Input: part model. Units: mm. Frame: model coordinates. Round coordinates to 2 decimals unless told otherwise and drop trailing zeros. Order: outer loops, then holes, each group sorted by start corner. A loop starts at its lowest first (then second) coordinate and runs counter-clockwise, first axis right, second up.
Item 1: Line query: L1, parallel to Y at x = -9.5, z = 1.4; L2, parallel to Y at x = 52, z = -0.8; L3, parallel to X at y = 3, z = -0.35. Output: solid intervals per line, ascending.
Item 2: Cut plane D-D on y = -9.5. Output: boundary loops of the cut face in (x, z).
Item 3: Cut plane A-A on y = 57. Output: boundary loops of the cut face in (x, z).
Item 4: First-contact query: pin 1 (6 mm diameter, centred on x = -52, y = 57, fed in from -Z); pin 2 (4 mm diameter, centred on x = -52, y = -57, fed in from -Z). Flat tips, straight axial feed; report the tip coordinate or a pass-through.
Item 5: Cut plane B-B on z = 1.2. Output: boundary loops of the cut face in (x, y), then the cut area to 3 significant figures.
Item 6: Cut plane C-C on x = 52. Output: boundary loops of the cut face in (y, z).
```python
from build123d import *

# Parameters (mm, degrees)
BOSS_EXTRUDE1_DEPTH         = 2
BOSS_EXTRUDE1_DEPTH_BACK    = 2
SKETCH1_W                   = 130
SKETCH1_H                   = 130
TAP_DRILL_FOR_M5X0_8_TAP1_D = 5
SKETCH5_W                   = 50
SKETCH5_H                   = 25
CUT_EXTRUDE2_DEPTH          = 20


with BuildPart() as part:
    # Sketch1 → Boss-Extrude1 (new, two sides: drawn at the far end of the back side and taken through both)
    with BuildSketch(Plane.XY.offset(-BOSS_EXTRUDE1_DEPTH_BACK)):
        Rectangle(SKETCH1_W, SKETCH1_H)
    extrude(amount=BOSS_EXTRUDE1_DEPTH + BOSS_EXTRUDE1_DEPTH_BACK)

    # Tap Drill for M5x0.8 Tap1 (through all)
    with Locations(Plane(origin=(0, 0, -2), x_dir=(-1, 0, 0), z_dir=(0, 0, -1))):
        with Locations((-52, 57), (52, 57), (52, -57), (-52, -57)):
            Hole(TAP_DRILL_FOR_M5X0_8_TAP1_D / 2)

    # Sketch5 → Cut-Extrude2 (cut)
    with BuildSketch(Plane(origin=(0, 0, -2), x_dir=(-1, 0, 0), z_dir=(0, 0, -1))):
        Rectangle(SKETCH5_W, SKETCH5_H)
    extrude(amount=-CUT_EXTRUDE2_DEPTH, mode=Mode.SUBTRACT)


solid = part.part
```
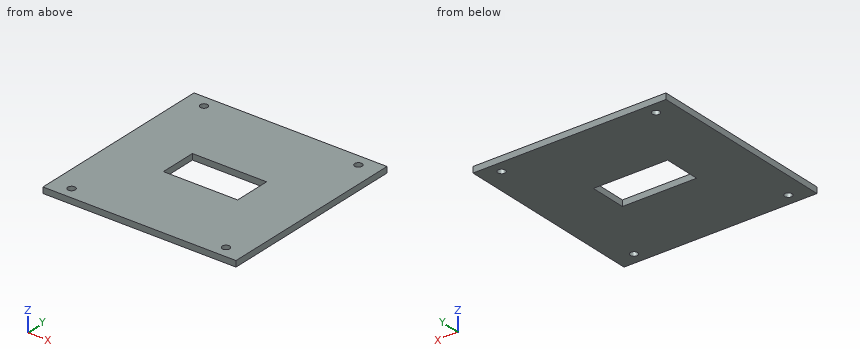
From the geometry:
1. L1: y = -65 to -12.5, 12.5 to 65
1. L2: y = -65 to -59.5, -54.5 to 54.5, 59.5 to 65
1. L3: x = -65 to -25, 25 to 65
2. outline: (-65, -2) - (-25, -2) - (-25, 2) - (-65, 2) - close; (25, -2) - (65, -2) - (65, 2) - (25, 2) - close
3. outline: (-65, -2) - (-54.5, -2) - (-54.5, 2) - (-65, 2) - close; (-49.5, -2) - (49.5, -2) - (49.5, 2) - (-49.5, 2) - close; (54.5, -2) - (65, -2) - (65, 2) - (54.5, 2) - close
4. pin 1: stops at z = -2
4. pin 2: passes through
5. outline: (-65, -65) - (65, -65) - (65, 65) - (-65, 65) - close; hole circle Ø5 at (-52, -57); hole circle Ø5 at (-52, 57); hole (-25, -12.5) - (25, -12.5) - (25, 12.5) - (-25, 12.5) - close; hole circle Ø5 at (52, -57); hole circle Ø5 at (52, 57)
5. area: 15,600 mm2
6. outline: (-65, -2) - (-59.5, -2) - (-59.5, 2) - (-65, 2) - close; (-54.5, -2) - (54.5, -2) - (54.5, 2) - (-54.5, 2) - close; (59.5, -2) - (65, -2) - (65, 2) - (59.5, 2) - close
